Geometry: see drawing. Coordinates: mm, zero at the bounding-box minimum. Round coordinates to 2 decimals unless told otherwise and drop trailing zeros. Order: outer loops, then holes, each group sorted by start corner. A loop starts at its lowest first (then second) coordinate and runs counter-clockwise, first axis right, second up.
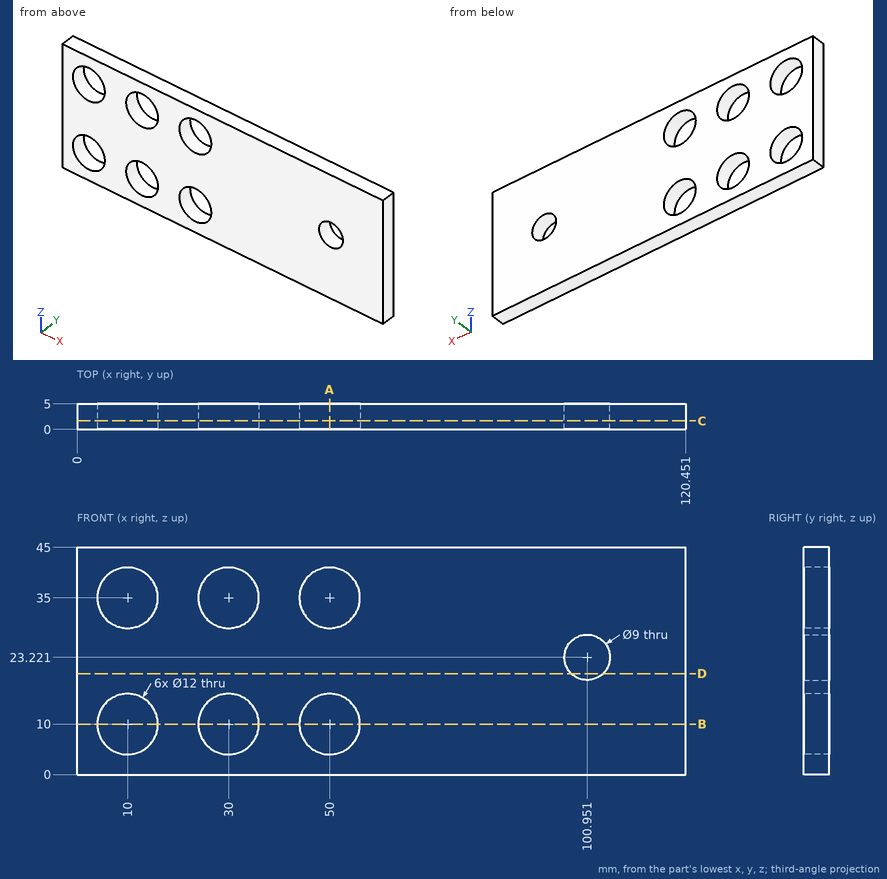
1. First-contact query: pin 1 (9.5 mm diameter, centred on x = 10, z = 35, fed in from -Y); pin 2 (1 mm diameter, centred on y = 1.5, z = 5, fed in from -X). Flat tips, straight axial feed; report the tip coordinate or a pass-through.
2. Section B-B on z = 10. Return loops of the section in (x, y).
3. Section A-A on x = 50. Return loops of the section in (y, z).
4. Section C-C on y = 1.65. Return loops of the section in (x, z), plus the area to 3 significant figures.
5. Section D-D on z = 20. Return loops of the section in (x, y), plus the area to 3 significant figures.
6. Line query: line 1 along Z through (x, y) = (29.5, 1.7); line 2 along X through (y, z) = (3.45, 10); line 3 along X through (y, z) = (2.35, 34). Output: solid intervals per line, ascending.
Result:
1. pin 1: passes through
1. pin 2: stops at x = 0
2. outline: (0, 0) - (4, 0) - (4, 5) - (0, 5) - close; (16, 0) - (24, 0) - (24, 5) - (16, 5) - close; (36, 0) - (44, 0) - (44, 5) - (36, 5) - close; (56, 0) - (120.45, 0) - (120.45, 5) - (56, 5) - close
3. outline: (0, 0) - (5, 0) - (5, 4) - (0, 4) - close; (0, 16) - (5, 16) - (5, 29) - (0, 29) - close; (0, 41) - (5, 41) - (5, 45) - (0, 45) - close
4. outline: (0, 0) - (120.45, 0) - (120.45, 45) - (0, 45) - close; hole circle Ø12 at (10, 10); hole circle Ø12 at (10, 35); hole circle Ø12 at (30, 10); hole circle Ø12 at (30, 35); hole circle Ø12 at (50, 10); hole circle Ø12 at (50, 35); hole circle Ø9 at (100.95, 23.22)
4. area: 4,680 mm2
5. outline: (0, 0) - (97.81, 0) - (97.81, 5) - (0, 5) - close; (104.09, 0) - (120.45, 0) - (120.45, 5) - (104.09, 5) - close
5. area: 571 mm2
6. line 1: z = 0 to 4.02, 15.98 to 29.02, 40.98 to 45
6. line 2: x = 0 to 4, 16 to 24, 36 to 44, 56 to 120.45
6. line 3: x = 0 to 4.08, 15.92 to 24.08, 35.92 to 44.08, 55.92 to 120.45
